from build123d import *

# Parameters (mm, degrees)
SKETCH_1_W               = 140
SKETCH_1_H               = 40
EXTRUDE_1_DEPTH          = 35
EXTRUDE_2_DEPTH          = 25
SKETCH_3_W               = 140
SKETCH_3_H               = 40
CUT_EXTRUDE_1_DEPTH      = 35
CUT_EXTRUDE_3_DEPTH      = 35
CUT_EXTRUDE_3_DEPTH_BACK = 35
CUT_EXTRUDE_4_DEPTH      = 35
CUT_EXTRUDE_4_DEPTH_BACK = 35
SKETCH_7_R               = 8.5
EXTRUDE_3_DEPTH          = 46
SKETCH_8_R               = 5
CUT_EXTRUDE_5_DEPTH      = 5


# Read off the part's stored shape, not the designer's step: 凸台-拉伸2
with BuildPart() as part:
    # 草图1 → 凸台-拉伸1 (new body)
    with BuildSketch(Plane.XY):
        Rectangle(SKETCH_1_W, SKETCH_1_H)
    extrude(amount=EXTRUDE_1_DEPTH)

    # 凸台-拉伸2 outline → 凸台-拉伸2 (add)
    with BuildSketch(Plane.XY.offset(35)):
        with BuildLine():
            add(Edge.make_bspline(
                [(4.99979571, 5.544461103), (14.93503193, -0.57740686), (21.362876996, 8.324395915)],
                knots=[6.93e-07, 6.93e-07, 6.93e-07, 1, 1, 1], degree=2))
            add(Edge.make_bspline(
                [(-62.204901581, 6.84122677), (-61.92798769, 6.977283921), (-60.294583456, 7.758325304), (-55.702877861, 9.628058542), (-47.815957259, 11.775440787), (-37.533060807, 13.26503558), (-26.917650518, 13.670745136), (-16.380744799, 12.945092857), (-6.360189442, 10.9325016), (0.253451635, 8.349640422), (3.857061157, 6.27680637), (4.666883474, 5.764061136), (4.99979571, 5.544461103)],
                knots=[0.117295231, 0.117295231, 0.117295231, 0.117295231, 0.129103067, 0.186305898, 0.302547913, 0.418789927, 0.535031942, 0.651273956, 0.767515971, 0.883757985, 0.904141366, 0.918671815, 0.918671815, 0.918671815, 0.918671815], degree=3))
            ThreePointArc((-62.204901581, 6.84122677), (-64.244084584, 4.997077414), (-65, 2.353642897))
            Line((-65, 2.353642897), (-65, 0.938055763))
            ThreePointArc((-65, 0.938055763), (-63.904973445, -0.928026304), (-61.741817309, -0.882190007))
            add(Edge.make_bspline(
                [(-61.741817309, -0.882190007), (-54.274901725, 3.714814791), (-28.022038825, 9.247775757), (-1.769175925, 3.780623693), (5, -3.520342201)],
                knots=[0.070063884, 0.070063884, 0.070063884, 0.070063884, 0.5, 1, 1, 1, 1], degree=3))
            add(Edge.make_bspline(
                [(5, -3.520342201), (12.391425527, -12.533975981), (37.865765315, -15.442874495), (40.911305501, 0)],
                knots=[0, 0, 0, 0, 1, 1, 1, 1], degree=3))
            add(Edge.make_bspline(
                [(40.911305501, 0), (41.685623973, 6.326172477), (33.243695942, 12.959768139), (23.757997073, 10.791133007), (21.362876996, 8.324395915)],
                knots=[0.14862794, 0.14862794, 0.14862794, 0.14862794, 0.452578319, 0.661483353, 0.661483353, 0.661483353, 0.661483353], degree=3))
        make_face()
    extrude(amount=EXTRUDE_2_DEPTH)

    # 草图3 → 切除-拉伸1 (cut)
    with BuildSketch(Plane(origin=(0, 0, 0), x_dir=(-1, 0, 0), z_dir=(0, 0, -1))):
        Rectangle(SKETCH_3_W, SKETCH_3_H)
    extrude(amount=-CUT_EXTRUDE_1_DEPTH, mode=Mode.SUBTRACT)

    # 草图4 → 切除-拉伸3 (cut, two sides: drawn at the far end of the back side and taken through both)
    with BuildSketch(Plane(origin=(0, 0, 0), x_dir=(1, 0, 0), z_dir=(0, 1, 0)).offset(-CUT_EXTRUDE_3_DEPTH_BACK)):
        with BuildLine():
            Line((40.990847483, -57), (-56, -57))
            add(Edge.make_bspline(
                [(-60.349653835, -60), (-58.152730496, -59.93219396), (-56, -57)],
                knots=[0.511562339, 0.511562339, 0.511562339, 1, 1, 1], degree=2))
            Line((-60.349653835, -60), (40.990847483, -60))
            Line((40.990847483, -60), (40.990847483, -57))
        make_face()
        with BuildLine():
            Line((-65, -60), (-60.557775934, -60))
            add(Edge.make_bspline(
                [(-65, -57), (-62.756791546, -59.93219396), (-60.557775934, -60)],
                knots=[0, 0, 0, 0.488437661, 0.488437661, 0.488437661], degree=2))
            Line((-65, -57), (-65, -60))
        make_face()
    extrude(amount=CUT_EXTRUDE_3_DEPTH + CUT_EXTRUDE_3_DEPTH_BACK, mode=Mode.SUBTRACT)

    # 草图6 → 切除-拉伸4 (cut, two sides: drawn at the far end of the back side and taken through both)
    with BuildSketch(Plane(origin=(0, 0, 0), x_dir=(1, 0, 0), z_dir=(0, 1, 0)).offset(-CUT_EXTRUDE_4_DEPTH_BACK)):
        with BuildLine():
            Line((40.990847483, -35), (21.362876991, -35))
            Line((21.362876991, -35), (-53.242217102, -35))
            add(Edge.make_bspline(
                [(40.990847483, -39), (-6.258890193, -46.635238136), (-53.242217102, -35)],
                knots=[0, 0, 0, 1, 1, 1], degree=2))
            Line((40.990847483, -39), (40.990847483, -35))
        make_face()
        with BuildLine():
            Line((-65, -36.715937701), (-63.25720797, -36.715937701))
            ThreePointArc((-63.25720797, -36.715937701), (-61.794491028, -36.60838225), (-60.363238722, -36.288029531))
            add(Edge.make_bspline(
                [(-60.363238722, -36.288029531), (-58.81156844, -35.818906777), (-57.248394022, -35.38946773), (-55.674749287, -35)],
                knots=[0.228745815, 0.228745815, 0.228745815, 0.228745815, 1, 1, 1, 1], degree=3))
            Line((-55.674749287, -35), (-65, -35))
            Line((-65, -35), (-65, -36.715937701))
        make_face()
    extrude(amount=CUT_EXTRUDE_4_DEPTH + CUT_EXTRUDE_4_DEPTH_BACK, mode=Mode.SUBTRACT)

    # 草图7 → 凸台-拉伸3 (add)
    with BuildSketch(Plane.XY.offset(57)):
        with Locations((30.911305501, 1.597813248)):
            Circle(SKETCH_7_R)
    extrude(amount=-EXTRUDE_3_DEPTH)

    # 草图8 → 切除-拉伸5 (cut)
    with BuildSketch(Plane(origin=(0, 0, 11), x_dir=(-1, 0, 0), z_dir=(0, 0, -1))):
        with Locations((-30.911305501, 1.597813248)):
            Circle(SKETCH_8_R)
    extrude(amount=-CUT_EXTRUDE_5_DEPTH, mode=Mode.SUBTRACT)


solid = part.part
Can you work these out from the model? Positions are in its coordinate system, mm. A direction names the side the tool comes from. Give positions to 0.01 mm unless a question says otherwise; leave off trailing zeros. Loops run counter-clockwise (first coordinate to the right, second up) from the corner with the lowest first, then second, coordinate; pieces in that order, holes last. Notation, with made-up numbers: (2.5, 40.5) -> (39.5, 40.5) arc R15 cw to (39.5, 58.5) -> close; hole circle Ø4 at (15, 31). An arc over 180 degrees is marked (long way). Return JSON: item names as keys, results as strings.
Q1. I want a section at A-A, the plane z = 21.5. List the corners of the cut face in (x, y) for me, then the cut area to 3 significant figures.
Checks:
{"outline": "circle Ø17 at (30.91, 1.6)", "area": "227 mm2"}
Q2. On a 3-axis mill with a long thin cutter (end or side, diameter ignored), from which of +Z, -Z, +X, -X, +Y, -Y can I reach the whole of each face in a straight line? I mean faces 1 (the face through (-54, 6, 35)), 2 (the face through (-64.223, 5.03, 47.945)), 3 (the face through (22.42, 1.97, 26.34)). Say none if no direction works.
Checks:
{"face 1": "-Z, -X, +Y, -Y", "face 2": "+Z, -Z, -X, +Y", "face 3": "-Z"}
Q3. We'd pull the mould along X, two halves only. Please class faces 4 (the face through (31, 2, 16)), 5 (the face through (3, 4, 57)), 6 (the face through (-61.81, 3.18, 36.61)): released by +X, released by -X, zero draft, split by the parting line, or undercut.
Checks:
{"face 4": "undercut", "face 5": "zero draft", "face 6": "released by -X"}
Q4. For pin 1 Ø3 at (x, y) = (25.5, 6.5) entering from +Z; pin 2 Ø1.9 at (x, y) = (-55, 5.5) entering from -Z; pin 3 Ø8 at (y, z) = (2.5, 19) entering from +X, each with a flat end and sliding along its axis, tell me the tip position at first contact or that it passes through.
Checks:
{"pin 1": "stops at z = 57", "pin 2": "stops at z = 35", "pin 3": "stops at x = 39.41"}
Q5. I need wall thicknesses on probe 1 along Z at (x, y) = (30.5, -4); probe 2 along Y at (x, z) = (-26.5, 55.5); probe 3 along Z at (x, y) = (28.5, 4.75). Which ranges of each line are inside material? Lowest first, please.
Checks:
{"probe 1": "z = 11 to 57", "probe 2": "y = 6.47 to 13.47", "probe 3": "z = 16 to 57"}
